For this review, take the finished solid that the model builds, in its own axes (mm). A direction names the side the tool comes from. Give positions to 0.01 mm unless a question says otherwise; leave off trailing zeros. Loops run counter-clockwise (first coordinate to the right, second up) from the corner with the lowest first, then second, coordinate; pieces in that order, holes last. Notation, with made-up numbers: (52, -11) -> (103, -11) arc R10 cw to (103, -5) -> close; hole circle Ø10 at (42.5, 61.25). An arc over 180 degrees is marked (long way). Write each question's results on one line, items separated by ' | '. Start each with the question number.
```python
from build123d import *

# Parameters (mm, degrees)
SKETCH2_R               = 10
SKETCH2_R_2             = 1.5
SKETCH2_R_3             = 0.736643129
SKETCH2_R_4             = 0.75
BOSS_EXTRUDE1_DEPTH     = 5
SKETCH3_R               = 10
BOSS_EXTRUDE2_DEPTH     = 15
SKETCH4_W               = 6
SKETCH4_H               = 10
CUT_EXTRUDE1_DEPTH      = 20
CUT_EXTRUDE1_DEPTH_BACK = 20
SKETCH5_R               = 3
CUT_EXTRUDE2_DEPTH      = 20
CUT_EXTRUDE2_DEPTH_BACK = 20


with BuildPart() as part:
    # Sketch2 → Boss-Extrude1 (new body)
    with BuildSketch(Plane.XY):
        Circle(SKETCH2_R)
        Circle(SKETCH2_R_2, mode=Mode.SUBTRACT)
        with Locations((7, 3)):
            Circle(SKETCH2_R_3, mode=Mode.SUBTRACT)
        with Locations((7, 0)):
            Circle(SKETCH2_R_4, mode=Mode.SUBTRACT)
        with Locations((7, -3)):
            Circle(SKETCH2_R_4, mode=Mode.SUBTRACT)
        with Locations((3, -7)):
            Circle(SKETCH2_R_4, mode=Mode.SUBTRACT)
        with Locations((0, -7)):
            Circle(SKETCH2_R_4, mode=Mode.SUBTRACT)
        with Locations((-3, -7)):
            Circle(SKETCH2_R_4, mode=Mode.SUBTRACT)
        with Locations((-7, -3)):
            Circle(SKETCH2_R_4, mode=Mode.SUBTRACT)
        with Locations((-7, 0)):
            Circle(SKETCH2_R_4, mode=Mode.SUBTRACT)
        with Locations((-7, 3)):
            Circle(SKETCH2_R_4, mode=Mode.SUBTRACT)
        with Locations((-3, 7)):
            Circle(SKETCH2_R_4, mode=Mode.SUBTRACT)
        with Locations((0, 7)):
            Circle(SKETCH2_R_4, mode=Mode.SUBTRACT)
        with Locations((3, 7)):
            Circle(SKETCH2_R_4, mode=Mode.SUBTRACT)
    extrude(amount=BOSS_EXTRUDE1_DEPTH)

    # Sketch3 → Boss-Extrude2 (add)
    with BuildSketch(Plane.XY):
        Circle(SKETCH3_R)
    extrude(amount=-BOSS_EXTRUDE2_DEPTH)

    # Sketch4 → Cut-Extrude1 (cut, two sides)
    with BuildSketch(Plane(origin=(0, 0, 0), x_dir=(1, 0, 0), z_dir=(0, 1, 0))) as cut_extrude1_sk:
        with Locations((0, 6.167476411)):
            Rectangle(SKETCH4_W, SKETCH4_H)
    extrude(amount=CUT_EXTRUDE1_DEPTH, mode=Mode.SUBTRACT)
    extrude(cut_extrude1_sk.sketch, amount=-CUT_EXTRUDE1_DEPTH_BACK, mode=Mode.SUBTRACT)

    # Sketch5 → Cut-Extrude2 (cut, two sides)
    with BuildSketch(Plane(origin=(0, 0, 0), x_dir=(0, 0, -1), z_dir=(1, 0, 0))) as cut_extrude2_sk:
        with Locations((6.167476411, 0)):
            Circle(SKETCH5_R)
    extrude(amount=CUT_EXTRUDE2_DEPTH, mode=Mode.SUBTRACT)
    extrude(cut_extrude2_sk.sketch, amount=-CUT_EXTRUDE2_DEPTH_BACK, mode=Mode.SUBTRACT)


solid = part.part
```
1. Draft analysis for pull direction Y (two halves, no side actions). For faces 4 (the flat face through (0, 7, 0)), 5 (the flat face through (0, 0, -15)), 6 (the flat face through (7, 3, 0)), state which applies: released by +Y, released by -Y, zero draft, split by the parting line, or undercut.
2. We need section C-C (y = 0). Write out the cut boundary in (x, z).
3. We need section B-B (z = -5.25). Write out the cut boundary in (x, y), plus the area to 3 significant figures.
4. Machinability: for faces 1 (the flat face through (0, -2, 5)), 2 (the flat face through (0, 0, -11.167)), 3 (the flat face through (3, -7, 0)), which of the approach directions +Z, -Z, +X, -X, +Y, -Y give a long, thin tool a straight path to every point of the face, cutting with its end or side? Answer none if there is none.
5. We need section A-A (x = 0). Write out the cut boundary in (y, z), plus the area to 3 significant figures.
6. For pin 1 Ø0.8 at (x, y) = (3, 7) entering from +Z; pin 2 Ø12 at (y, z) = (7, -5) entering from +X; pin 3 Ø2 at (x, z) = (6, -6) entering from +Y, all flat-tipped, find the tip position at first contact; note any pin that passes through.
7. Wall thickness on L1, parallel to Y at x = 3, z = 2.1; L2, parallel to Z at x = 8.25, y = 0; L3, parallel to Y at x = 7, z = 1.9: over which ranges is each line inside the solid? List them lowest first.
8. We need section D-D (y = 5.25). Write out the cut boundary in (x, z), plus the area to 3 significant figures.
Response:
1) face 4: undercut | face 5: zero draft | face 6: undercut
2) outline: (-10, -15) -> (10, -15) -> (10, -9.17) -> (3, -9.17) -> (3, -11.17) -> (-3, -11.17) -> (-3, -9.17) -> (-10, -9.17) -> close; (-10, -3.17) -> (-3, -3.17) -> (-3, -1.17) -> (3, -1.17) -> (3, -3.17) -> (10, -3.17) -> (10, 5) -> (7.75, 5) -> (7.75, 0) -> (6.25, 0) -> (6.25, 5) -> (1.5, 5) -> (1.5, 0) -> (-1.5, 0) -> (-1.5, 5) -> (-6.25, 5) -> (-6.25, 0) -> (-7.75, 0) -> (-7.75, 5) -> (-10, 5) -> close
3) outline: (-9.58, -2.86) arc R10 ccw to (-3, -9.54) -> (-3, -2.86) -> close; (-9.58, 2.86) -> (-3, 2.86) -> (-3, 9.54) arc R10 ccw to start; (3, -9.54) arc R10 ccw to (9.58, -2.86) -> (3, -2.86) -> close; (3, 2.86) -> (9.58, 2.86) arc R10 ccw to (3, 9.54) -> close | area: 118 mm2
4) face 1: +Z, +X, -X, +Y, -Y | face 2: +Y, -Y | face 3: +Z
5) outline: (-10, -15) -> (10, -15) -> (10, -11.17) -> (-10, -11.17) -> close; (-10, -1.17) -> (10, -1.17) -> (10, 5) -> (7.75, 5) -> (7.75, 0) -> (6.25, 0) -> (6.25, 5) -> (1.5, 5) -> (1.5, 0) -> (-1.5, 0) -> (-1.5, 5) -> (-6.25, 5) -> (-6.25, 0) -> (-7.75, 0) -> (-7.75, 5) -> (-10, 5) -> close | area: 170 mm2
6) pin 1: stops at z = 0 | pin 2: stops at x = 9.93 | pin 3: stops at y = 8.66
7) L1: y = -9.54 to -7.75, -6.25 to 6.25, 7.75 to 9.54 | L2: z = -15 to -9.17, -3.17 to 5 | L3: y = -7.14 to -3.75, -2.25 to -0.75, 0.75 to 2.26, 3.74 to 7.14
8) outline: (-8.51, -15) -> (8.51, -15) -> (8.51, 5) -> (-8.51, 5) -> close; hole (-3, -11.17) -> (3, -11.17) -> (3, -1.17) -> (-3, -1.17) -> close | area: 280 mm2
